from build123d import *

# Parameters (mm, degrees)
SKETCH_2_R               = 2.2
SKETCH_2_R_2             = 1.55
CUT_EXTRUDE_1_DEPTH      = 47.584117465
PATTERN_CIRCULAR_1_COUNT = 4


with BuildPart() as part:
    # 草图1 → 旋转1 (revolve)
    with BuildSketch(Plane.XY, mode=Mode.PRIVATE) as revolve_1_sk:
        Polygon((0, 0), (25.2, 0), (25.2, 30), (23, 30), (23, 2.2), (0, 2.2), align=None)
    revolve(revolve_1_sk.sketch.rotate(Axis((0, 2.2, 0), (0, -1, 0)), 90), axis=Axis((0, 2.2, 0), (0, -1, 0)))

    # 草图2 → 切除-拉伸1 (cut, through all)
    with BuildSketch(Plane.XZ):
        with Locations(Location((0, 0, 0), (0, 0, 270))):
            Circle(SKETCH_2_R)
        with Locations(Location((8.5, 0, 0), (0, 0, 270))):
            Circle(SKETCH_2_R_2)
    cut_extrude_1 = extrude(amount=-CUT_EXTRUDE_1_DEPTH, mode=Mode.SUBTRACT)

    # 阵列(圆周)1: 切除-拉伸1 ×4 about axis
    pattern_circular_1_axis = Axis((0, 0, 0), (0, 1, 0))
    for i in range(1, PATTERN_CIRCULAR_1_COUNT):
        add(cut_extrude_1.rotate(pattern_circular_1_axis, i * 360 / PATTERN_CIRCULAR_1_COUNT), mode=Mode.SUBTRACT)


solid = part.part
Check sheet for the modelled part. Datum: model origin and axes. Units: mm. A direction names the side the tool comes from. Round coordinates to 2 decimals unless told otherwise and drop trailing zeros. Write each loop counter-clockwise with the first axis right and the second up, starting at its lowest first coordinate (ties: lowest second). Pieces come first, ordered by that corner, then holes. Notation, with made-up numbers: (59, -8.75) - (102, -8.75) arc R25 ccw to (102, 12.25) - close; hole circle Ø10 at (67, 18.5). An arc over 180 degrees is marked (long way). Return JSON: item names as keys, results as strings.
Q1. Scan lines: L1, parallel to X at y = 1.55, z = 0; L2, parallel to Z at x = -0.5, y = 2.5; L3, parallel to Y at x = 6, z = -3.5. Record each from-to range of solid material in increasing order. Write a range as from..to.
Returned:
{"L1": "x = -25.2..-10.05, -6.95..-2.2, 2.2..6.95, 10.05..25.2", "L2": "z = -25.2..-22.99, 22.99..25.2", "L3": "y = 0..2.2"}
Q2. Access from +Z, -Z, +X, -X, +Y, -Y to the whole of each face (thin tool, end or side, straight path). Record for faces 4 (the cylindrical face through (6.987, 1.085, 0.336)), 5 (the flat face through (0, 2.2, 5)).
Returned:
{"face 4": "+Y, -Y", "face 5": "+Y"}
Q3. Cross-section at B-B (z = 0). Record the boundary of the cut face in (x, y).
Returned:
{"outline": "(-25.2, 0) - (-10.05, 0) - (-10.05, 2.2) - (-23, 2.2) - (-23, 30) - (-25.2, 30) - close; (-6.95, 0) - (-2.2, 0) - (-2.2, 2.2) - (-6.95, 2.2) - close; (2.2, 0) - (6.95, 0) - (6.95, 2.2) - (2.2, 2.2) - close; (10.05, 0) - (25.2, 0) - (25.2, 30) - (23, 30) - (23, 2.2) - (10.05, 2.2) - close"}
Q4. Cross-section at D-D (x = 22). Record the boundary of the cut face in (y, z), then the cut area to 3 significant figures.
Returned:
{"outline": "(0, -12.29) - (30, -12.29) - (30, -6.71) - (2.2, -6.71) - (2.2, 6.71) - (30, 6.71) - (30, 12.29) - (0, 12.29) - close", "area": "364 mm²"}
Q5. Cross-section at A-A (x = 0). Record the boundary of the cut face in (y, z).
Returned:
{"outline": "(0, -25.2) - (30, -25.2) - (30, -23) - (2.2, -23) - (2.2, -10.05) - (0, -10.05) - close; (0, -6.95) - (2.2, -6.95) - (2.2, -2.2) - (0, -2.2) - close; (0, 2.2) - (2.2, 2.2) - (2.2, 6.95) - (0, 6.95) - close; (0, 10.05) - (2.2, 10.05) - (2.2, 23) - (30, 23) - (30, 25.2) - (0, 25.2) - close"}
Q6. Draft check along Z on faces 1 (the flat face through (20.4, 30, 11.1)), 2 (the cylindrical face through (15.33, 15.21, -20)), 3 (the cylindrical face through (-22.804, 15.905, -2.994)). Enter one of: released by +Z, released by -Z, zero draft, split by the parting line, or undercut.
Returned:
{"face 1": "zero draft", "face 2": "split by the parting line", "face 3": "undercut"}
Q7. Cross-section at C-C (z = -8.5). Record the boundary of the cut face in (x, y), then the cut area to 3 significant figures.
Returned:
{"outline": "(-23.72, 0) - (-1.55, 0) - (-1.55, 2.2) - (-21.37, 2.2) - (-21.37, 30) - (-23.72, 30) - close; (1.55, 0) - (23.72, 0) - (23.72, 30) - (21.37, 30) - (21.37, 2.2) - (1.55, 2.2) - close", "area": "228 mm²"}
Q8. Depth check by flat-ended pin: P1, Ø5, axis at x = 8.5, z = 0, coming from the +Y side; P2, Ø4, axis at x = 0, z = 0, coming from the +Y side; P3, Ø3, axis at x = 19, y = 10, coming from the -Z side; P4, Ø2, axis at y = 13.5, z = 14.5, coming from the -X side. Enter the tip coordinate at first touch or a pass-through.
Returned:
{"P1": "stops at y = 2.2", "P2": "passes through", "P3": "stops at z = -18.13", "P4": "stops at x = -21.28"}
